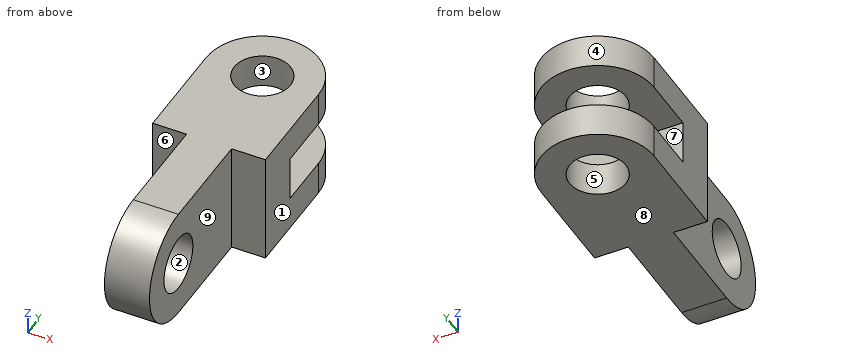
from build123d import *

# Parameters (mm, degrees)
CROQUIS1_R                   = 25
CROQUIS1_W                   = 100
CROQUIS1_H                   = 42
SALIENTE_EXTRUIR1_DEPTH      = 30
CROQUIS4_W                   = 100
CROQUIS4_H                   = 42
SALIENTE_EXTRUIR2_DEPTH      = 40
CROQUIS5_R                   = 25
SALIENTE_EXTRUIR3_DEPTH      = 30
SALIENTE_EXTRUIR4_DEPTH      = 20
SALIENTE_EXTRUIR4_DEPTH_BACK = 20
CROQUIS6_R                   = 25


with BuildPart() as part:
    # Croquis1 → Saliente-Extruir1 (new body)
    # profile 1 of 2: a face of its own
    with BuildSketch(Plane.XY):
        with BuildLine():
            ThreePointArc((50, 0), (0, 50), (-50, 0))
            Line((-50, 0), (-50, -50))
            Line((-50, -50), (50, -50))
            Line((50, -50), (50, 0))
        make_face()
        Circle(CROQUIS1_R, mode=Mode.SUBTRACT)
    # profile 2 of 2: a face of its own
    with BuildSketch(Plane.XY):
        with Locations((0, -71)):
            Rectangle(CROQUIS1_W, CROQUIS1_H)
    extrude(amount=-SALIENTE_EXTRUIR1_DEPTH)

    # Croquis4 → Saliente-Extruir2 (add)
    with BuildSketch(Plane(origin=(0, 0, -30), x_dir=(-1, 0, 0), z_dir=(0, 0, -1))):
        with Locations((0, -71)):
            Rectangle(CROQUIS4_W, CROQUIS4_H)
    extrude(amount=SALIENTE_EXTRUIR2_DEPTH)

    # Croquis5 → Saliente-Extruir3 (add)
    with BuildSketch(Plane(origin=(0, 0, -70), x_dir=(-1, 0, 0), z_dir=(0, 0, -1))):
        with BuildLine():
            Line((-50, 0), (-50, -92))
            Line((-50, -92), (50, -92))
            Line((50, -92), (50, 0))
            ThreePointArc((50, 0), (0, 50), (-50, 0))
        make_face()
        with Locations(Location((0, 0, 0), (0, 0, 180))):
            Circle(CROQUIS5_R, mode=Mode.SUBTRACT)
    extrude(amount=SALIENTE_EXTRUIR3_DEPTH)

    # Croquis6 → Saliente-Extruir4 (add, two sides: drawn at the far end of the back side and taken through both)
    with BuildSketch(Plane(origin=(0, 0, 0), x_dir=(0, 0, -1), z_dir=(1, 0, 0)).offset(-SALIENTE_EXTRUIR4_DEPTH_BACK)):
        with BuildLine():
            Line((0, -184), (0, -92))
            Line((0, -92), (100, -92))
            Line((100, -92), (100, -184))
            ThreePointArc((100, -184), (50, -234), (0, -184))
        make_face()
        with Locations((50, -184)):
            Circle(CROQUIS6_R, mode=Mode.SUBTRACT)
    extrude(amount=SALIENTE_EXTRUIR4_DEPTH + SALIENTE_EXTRUIR4_DEPTH_BACK)


solid = part.part
For this review, take the finished solid that the model builds, in its own axes (mm). Face numbers are marked on the shaded views. A direction names the side the tool comes from. Round coordinates to 2 decimals unless told otherwise and drop trailing zeros. Write each loop counter-clockwise with the first axis right and the second up, starting at its lowest first coordinate (ties: lowest second). Pieces come first, ordered by that corner, then holes. Notation, with made-up numbers: (-2, 56.5) -> (25, 56.5) arc R28 ccw to (25, 90.5) -> close; hole circle Ø3 at (71.5, 2.5). An arc over 180 degrees is marked (long way). Put each result on its own line as item: value.
Q1. Consider section A-A on x = 0. State the section outline as (y, z) points.
Determined:
outline: (-184, -100) -> (-25, -100) -> (-25, -70) -> (-50, -70) -> (-50, -30) -> (-25, -30) -> (-25, 0) -> (-184, 0) arc R50 ccw to start; (25, -100) -> (50, -100) -> (50, -70) -> (25, -70) -> close; (25, -30) -> (50, -30) -> (50, 0) -> (25, 0) -> close; hole circle Ø50 at (-184, -50)
Q2. Consider section B-B on z = -50. State the section outline as (x, y) points, and give its area (3 significant figures).
Determined:
outline: (-50, -92) -> (-20, -92) -> (-20, -159) -> (20, -159) -> (20, -92) -> (50, -92) -> (50, -50) -> (-50, -50) -> close; (-20, -234) -> (20, -234) -> (20, -209) -> (-20, -209) -> close
area: 7,880 mm^2
Q3. Clearance check with flat-ended pins moving along their axes: pin 1 Ø2 at (x, z) = (-23.5, -66.5) entering from +Y; pin 2 Ø24 at (x, z) = (39.5, -64.5) entering from -Y; pin 3 Ø1 at (x, z) = (9, -56) entering from -Y. State where each tip first meets the part, or that it passes through.
Determined:
pin 1: stops at y = -50
pin 2: stops at y = -92
pin 3: stops at y = -233.7
Q4. Machinability: for the marked faces 5, 6, 7, 8 and 9, which of the approach directions +Z, -Z, +X, -X, +Y, -Y give a long, thin tool a straight path to every point of the face, cutting with its end or side? Answer none if there is none.
Determined:
face 5: +Z, -Z
face 6: +Z, -Z, -X, -Y
face 7: +X, -X, +Y
face 8: -Z, +X, -X, +Y, -Y
face 9: +Z, -Z, +X, -Y
Q5. To check wall thickness, follow L1, parallel to Z at x = 41, y = 10.5; L2, parallel to X at y = -164.5, z = -71; L3, parallel to Y at x = -8.5, z = -50. State the ranges of each line that lie inside material, in increasing order. Write a range as [from, to].
Determined:
L1: z = [-100, -70], [-30, 0]
L2: x = [-20, 20]
L3: y = [-234, -209], [-159, -50]
Q6. Consider section C-C on y = 10.5. State the section outline as (x, z) points.
Determined:
outline: (-48.89, -100) -> (-22.69, -100) -> (-22.69, -70) -> (-48.89, -70) -> close; (-48.89, -30) -> (-22.69, -30) -> (-22.69, 0) -> (-48.89, 0) -> close; (22.69, -100) -> (48.89, -100) -> (48.89, -70) -> (22.69, -70) -> close; (22.69, -30) -> (48.89, -30) -> (48.89, 0) -> (22.69, 0) -> close
Q7. The part is to be moulded in two halves that separate along Y. For the marked faces 1, 2, 3 and 4, say which applies: released by +Y, released by -Y, zero draft, split by the parting line, or undercut.
Determined:
face 1: zero draft
face 2: undercut
face 3: undercut
face 4: released by +Y
Q8. Consider section D-D on z = -15.5. State the section outline as (x, y) points, and give its area (3 significant figures).
Determined:
outline: (-50, -92) -> (-20, -92) -> (-20, -220.19) -> (20, -220.19) -> (20, -92) -> (50, -92) -> (50, 0) arc R50 ccw to (-50, 0) -> close; hole circle Ø50 at (0, 0)
area: 16,300 mm^2
